Answer from the drawing. Dimensions are ordinates in mm from the lowest x, y and z of the part. A direction names the side the tool comes from. Give positions to 0.01 mm unless a question says otherwise; leave off trailing zeros. Order: outer loops, then holes, each group sorted by start corner. A loop starts at its lowest first (then second) coordinate and runs counter-clockwise, first axis right, second up. Notation, with made-up numbers: (43, 74.5) - (79, 74.5) arc R17 cw to (79, 85.5) - close; hole circle Ø11 at (22.5, -7). An arc over 180 degrees is marked (long way). Answer in a Markdown table with one row per item.
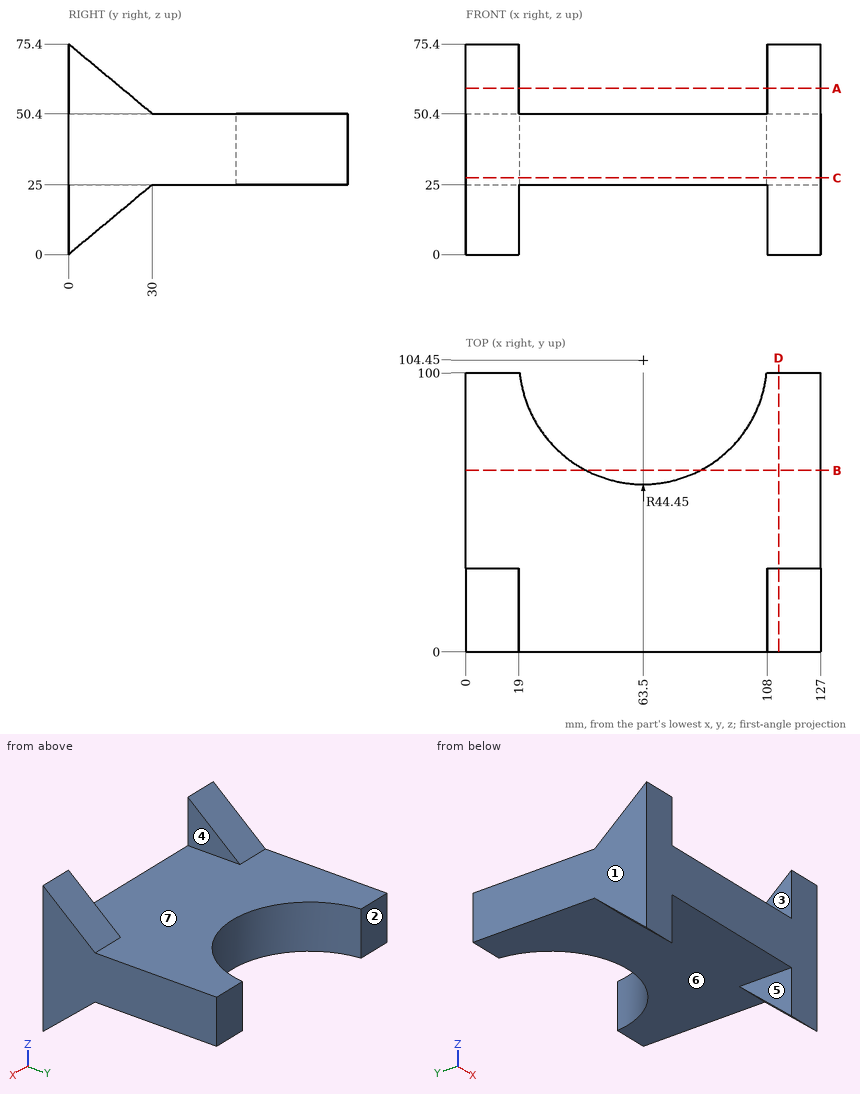
Item 1: Find section C-C on z = 27.5. Write down the section's boundary in (x, y), then the cut area to 3 significant figures.
Answer block:
| item | result |
|---|---|
| outline | (0, 0) - (127, 0) - (127, 100) - (107.73, 100) arc R44.45 cw to (19.27, 100) - (0, 100) - close |
| area | 9,990 mm² |
Item 2: Each of these flat-tipped pins is pushed along its axis until it touches: P1, Ø4, axis at x = 36.5, y = 64.5, coming from the -Z side; P2, Ø8, axis at x = 85, z = 48.5, coming from the +Y side; P3, Ø3, axis at x = 77.5, z = 33, coming from the +Y side. Where does it stop, or does it pass through?
Answer block:
| item | result |
|---|---|
| P1 | z = 25 |
| P2 | y = 68.04 |
| P3 | y = 62.79 |
Item 3: Consider line 1 (X direction, y = 5, z = 23.5); line 2 (Z direction, x = 77, y = 54); line 3 (X direction, y = 72, z = 28). Determine where each line is inside the solid, lowest interval first.
Answer block:
| item | result |
|---|---|
| line 1 | 0 to 19, 108 to 127 |
| line 2 | 25 to 50.4 |
| line 3 | 0 to 33.12, 93.88 to 127 |
Item 4: Find section D-D on x = 112. Write down the section's boundary in (y, z).
Answer block:
| item | result |
|---|---|
| outline | (0, 0) - (30, 25) - (100, 25) - (100, 50.4) - (30, 50.4) - (0, 75.4) - close |
Item 5: Determine the mould class of the marked faces 1, 2 and 3 for opening direction X: pulls with the +X half, pulls with the -X half, needs draft (parallel to the pull), parting line crosses it, or undercut.
Answer block:
| item | result |
|---|---|
| face 1 | pulls with the -X half |
| face 2 | needs draft |
| face 3 | undercut |
Item 6: Which of the six approach directions +Z, -Z, +X, -X, +Y, -Y give full straight-line access (tool end or side, diameter ignored) to the marked faces 4, 5, 6 and 7?
Answer block:
| item | result |
|---|---|
| face 4 | +Z, +Y, -Y |
| face 5 | -Z, +Y, -Y |
| face 6 | -Z, +Y |
| face 7 | +Z, +Y |
Item 7: Find section A-A on z = 59.5. Write down the section's boundary in (x, y), then the cut area to 3 significant figures.
Answer block:
| item | result |
|---|---|
| outline | (0, 0) - (19, 0) - (19, 19.08) - (0, 19.08) - close; (108, 0) - (127, 0) - (127, 19.08) - (108, 19.08) - close |
| area | 725 mm² |
Item 8: Find section B-B on y = 65. Write down the section's boundary in (x, z).
Answer block:
| item | result |
|---|---|
| outline | (0, 25) - (43.02, 25) - (43.02, 50.4) - (0, 50.4) - close; (83.98, 25) - (127, 25) - (127, 50.4) - (83.98, 50.4) - close |
